Part model, mm, in its own coordinate system. A direction names the side the tool comes from. Give positions to 0.01 mm unless a question says otherwise; leave off trailing zeros. Loops run counter-clockwise (first coordinate to the right, second up) from the corner with the lowest first, then second, coordinate; pieces in that order, holes last. Notation, with made-up numbers: (54, -29.5) -> (61, -29.5) arc R16 cw to (61, -13.5) -> close; hole circle Ø5 at (20.25, 62). An arc over 180 degrees is marked (long way). Write item = value, one per line.
Autodesk Inventor part; units mm, degrees
ref_plane "Plano de trabajo1" through (1.52, 1.52, 0.76) normal (0, 1, 0) x (0, 0, 1)
ref_plane "Plano de trabajo2" through (1.52, 1.52, 0.76) normal (1, 0, 0) x (0, 1, 0)
ref_plane "YZ Plane" through (0, 0, 0) normal (1, 0, 0) x (0, 1, 0)
sketch "Boceto1" plane through (0, 0, 0) normal (0, 0, 1) x (1, 0, 0)
  line L0 (0, 0) -> (385, 0)
  line L1 (385, 0) -> (385, 230)
  line L2 (385, 230) -> (0, 230)
  line L3 (0, 230) -> (0, 0)
  dimension "d0" = 385
  dimension "d1" = 230
extrude "Extrusión1" add sketch "Boceto1" along normal blind 0.91
sketch "Boceto2" plane through (0, 0, 0.91) normal (0, 0, 1) x (1, 0, 0)
  line L0 (385, 230) -> (0, 230)
  line L1 (0, 0) -> (0.76, 0)
  line L2 (0.91, 0.91) -> (0.91, 229.09)
  line L3 (0.91, 230) -> (0, 230)
  line L4 (0, 230) -> (0, 0)
  line L5 (0, 230) -> (0, 0)
  line L6 (385, 0) -> (385, 230)
  line L7 (0, 0) -> (385, 0)
  line L8 (385, 0) -> (385, 0.91)
  line L9 (384.09, 0.91) -> (0.91, 0.91)
  line L10 (0, 0.76) -> (0, 0)
  line L11 (0, 0) -> (385, 0)
  line L12 (385, 0) -> (384.24, 0)
  line L13 (384.09, 0.91) -> (384.09, 229.09)
  line L14 (384.09, 230) -> (385, 230)
  line L15 (385, 230) -> (385, 0)
  line L16 (385, 230) -> (0, 230)
  line L17 (0, 230) -> (0, 229.09)
  line L18 (0.91, 229.09) -> (384.09, 229.09)
  line L19 (385, 229.24) -> (385, 230)
  dimension "d36" = 0.91
  dimension "d37" = 0.91
  dimension "d38" = 0.91
  dimension "d39" = 0.91
extrude "Extrusión2" add sketch "Boceto2" along normal blind 20
sketch "Boceto3" plane through (0, 0, 0) normal (0, 0, -1) x (-1, 0, 0)
  line L0 (-384.09, 0.91) -> (-384.09, 229.09)
  line L1 (-0.91, 0.91) -> (-384.09, 0.91)
  line L2 (-365.39, 0.91) -> (-351.39, 0.91) construction
  circle A0 centre (-365.24, 14.76) radius 1
  line L3 (-385, 230) -> (-366, 230)
  line L4 (-385, 230) -> (0, 230)
  line L5 (-366, 230) -> (-366, 216)
  circle A1 centre (-366, 216) radius 1.5875
  line L6 (-366, 216) -> (-108, 216)
  circle A2 centre (-108, 216) radius 1.5875
  point P0 (0, 0)
  dimension "d14" = 19
  dimension "d15" = 14
  dimension "d16" = 90
  dimension "d17" = 3.175
  dimension "d18" = 258
  dimension "d19" = 3.175
extrude "Extrusión3" cut sketch "Boceto3" against normal through all contours A1 L6 L5 | A2 | L5 L6 A1
sketch "Boceto4" plane through (0, 0, 0) normal (0, -1, 0) x (1, 0, 0)
  line L0 (0, 0) -> (0, 20.91) construction
  line L1 (385, 0) -> (385, 20.91) construction
  line L2 (0, 10.455) -> (20, 10.455) construction
  circle A0 centre (20, 10.455) radius 2.5
  circle A1 centre (192.5, 10.455) radius 2.5
  circle A2 centre (365, 10.455) radius 2.5
  line L3 (384.09, 20.91) -> (0.91, 20.91)
  dimension "d25" = 5
  dimension "d26" = 5
  dimension "d27" = 5
  dimension "d41" = 20
  dimension "d42" = 20
ref_plane "Plano de trabajo1" through (1.52, 1.52, 0.76) normal (0, 1, 0) x (0, 0, 1)
extrude "Extrusión4" cut sketch "Boceto4" against normal up to surface (1.52 mm away)
sketch "Boceto5" plane through (0, 0, 0) normal (-1, 0, 0) x (0, 0, 1)
  line L0 (0, 0) -> (20.91, 0) construction
  line L1 (10.455, 0) -> (10.455, 230) construction
  line L2 (0, 230) -> (20.91, 230) construction
  line L3 (10.455, 0) -> (10.455, 40) construction
  line L4 (10.455, 230) -> (10.455, 190) construction
  circle A0 centre (10.455, 40) radius 2.5
  circle A1 centre (10.455, 190) radius 2.5
  dimension "d30" = 40
  dimension "d31" = 40
  dimension "d32" = 5
  dimension "d33" = 5
ref_plane "Plano de trabajo2" through (1.52, 1.52, 0.76) normal (1, 0, 0) x (0, 1, 0)
extrude "Extrusión5" cut sketch "Boceto5" against normal up to surface (1.52 mm away)
equation "\"d25\" = d27"
equation "\"d26\" = d27"
equation "\"d41\" = d42"
equation "\"d30\" = d31"
equation "\"d32\" = d33"
properties part number "Tapa_superior_derecha" material "Acero AISI 1006 85 LC"
1) Slice it at A-A, the plane y = 28. List the corners of the cut face in (x, z).
Resolved:
outline = (0, 0) -> (385, 0) -> (385, 20.91) -> (384.09, 20.91) -> (384.09, 0.91) -> (0.91, 0.91) -> (0.91, 20.91) -> (0, 20.91) -> close
2) Drop a flat-ended pin along its axis: P1, Ø3, axis at y = 190, z = 10.455, coming from the -X side. Give the stop position or say it passes through.
Resolved:
P1 = 384.09
3) Pull direction X, two halves, no side cores. Call faces 3 (the face through (385, 113, 10)), 4 (the face through (0, 117, 10)), 5 (the face through (384.09, 113, 11)), 6 (the face through (195, 230, 10)): pulls with the +X half, pulls with the -X half, needs draft (parallel to the pull), parting line crosses it, or undercut.
Resolved:
face_3 = pulls with the +X half
face_4 = pulls with the -X half
face_5 = undercut
face_6 = needs draft
4) Slice it at B-B, the plane x = 288. List the corners of the cut face in (y, z).
Resolved:
outline = (0, 0) -> (230, 0) -> (230, 20.91) -> (229.09, 20.91) -> (229.09, 0.91) -> (0.91, 0.91) -> (0.91, 20.91) -> (0, 20.91) -> close
5) Which spindle directions (+Z, -Z, +X, -X, +Y, -Y) get a long thin tool onto all of the face, cutting with end or side? Do faces 1 (the face through (190, 229.09, 11)), 2 (the face through (189.8, 0, 10.3)). Say none if no direction does.
Resolved:
face_1 = +Z
face_2 = +Z, -Z, +X, -X, -Y
6) Drill centre lines: line 1 along X through (y, z) = (205.5, 14); line 2 along Y through (x, z) = (353.5, 5.25); line 3 along X through (y, z) = (216, 0.4). Where is each one in solid material? Low to high. Write a range as [from, to].
Resolved:
line_1 = [0, 0.91], [384.09, 385]
line_2 = [0, 0.91], [229.09, 230]
line_3 = [0, 106.41], [109.59, 364.41], [367.59, 385]
